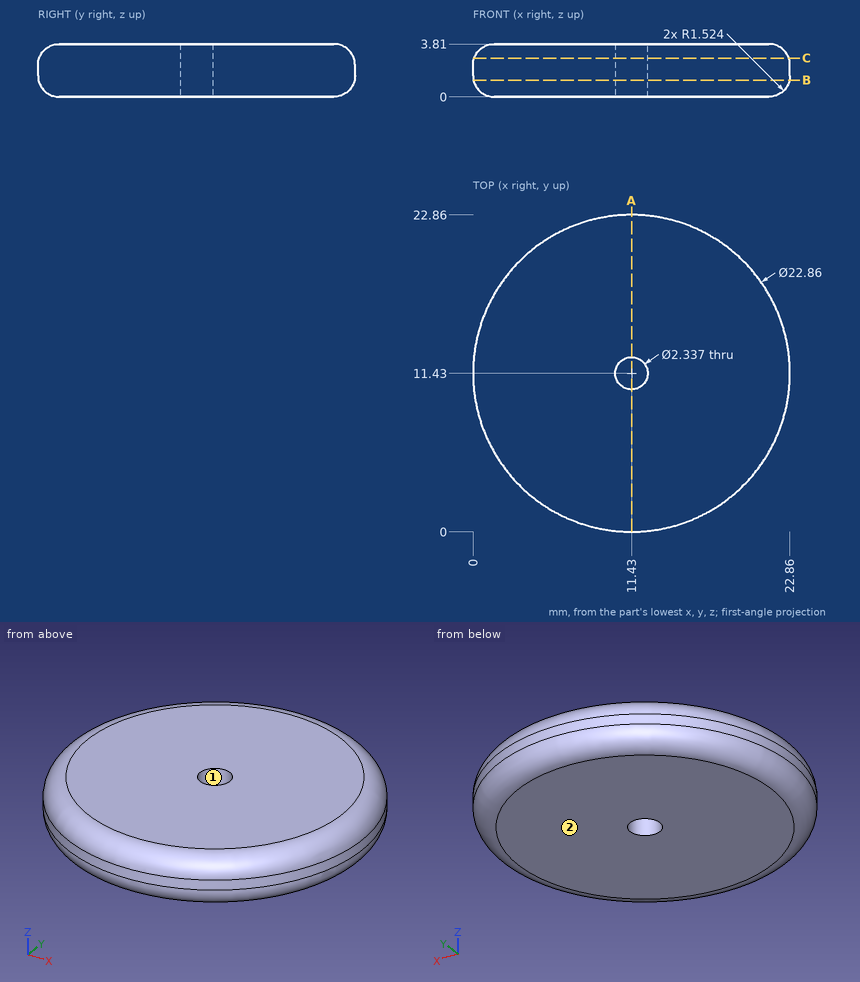
Drawing for the job (mm, zero at the part's lowest x, y, z). Give positions to 0.01 mm unless a question says otherwise; leave off trailing zeros. Loops run counter-clockwise (first coordinate to the right, second up) from the corner with the lowest first, then second, coordinate; pieces in that order, holes last. Notation, with made-up numbers: M 65,84 L 108,84 A17 ccw 108,99 Z; hole C 50.25,41.25 d10. An arc over 180 degrees is marked long. One line per question, with ' | ' between items. Start each with the question number.
1. Two-plate mould, pull along Y, no slides. Class the marked faces 1 and 2: pulls with the +Y half, pulls with the -Y half, needs draft (parallel to the pull), parting line crosses it, or undercut.
2. Flat gauge pin, fed straight in: pin 1 (1 mm diameter, centred on y = 10, z = 2, fed in from -X). Where does the tip first touch, or does it go through?
3. Probe L1, parallel to Y at x = 11.43, z = 1.9; L2, parallel to Y at x = 11.43, z = 2.85. List the from-to ranges inside material, lowest first. Write a range as from..to.
4. Saw through at A-A on x = 11.43. Give the cut face in (y, z), plus the area to 3 significant figures.
5. Saw through at B-B on z = 1.2. Give the cut face in (x, y) (1 decimal), plus the area to 3 significant figures.
6. Saw through at C-C on z = 2.8. Give the cut face in (x, y), plus the area to 3 significant figures.
Result sheet:
1) face 1: undercut | face 2: needs draft
2) pin 1: stops at x = 0.04
3) L1: y = 0..10.26, 12.6..22.86 | L2: y = 0.11..10.26, 12.6..22.75
4) outline: M 0,1.52 A1.52 ccw 1.52,0 L 10.26,0 L 10.26,3.81 L 1.52,3.81 A1.52 ccw 0,2.29 Z; M 12.6,0 L 21.34,0 A1.52 ccw 22.86,1.52 L 22.86,2.29 A1.52 ccw 21.34,3.81 L 12.6,3.81 Z | area: 76.2 mm^2
5) outline: C 11.4,11.4 d22.8; hole C 11.4,11.4 d2.3 | area: 404 mm^2
6) outline: C 11.43,11.43 d22.68; hole C 11.43,11.43 d2.34 | area: 400 mm^2
